Job drawing, mm, ordinate dimensions from the low corner. One solid piece. Coordinates: 2 decimals unless noted, no trailing zeros. Loops run counter-clockwise (first coordinate to the right, second up) from the corner with the lowest first, then second, coordinate; pieces in that order, holes last. Notation, with made-up numbers: (89, -31) - (112, -31) arc R24 ccw to (112, 4) - close; hole circle Ø4 at (32, 52.25). An arc over 180 degrees is marked (long way). Use a Markdown table: item, result. Add a question column.
1) Band-saw the part on B-B (y = 1.6). Give the cut face in (x, z), plus the area to 3 significant figures.
2) Band-saw the part on A-A (z = 5). Give the cut face in (x, y), plus the area to 3 significant figures.
3) Probe probe 1 along Z at (x, y) = (4.7, 1.3); probe 2 along X at (y, z) = (0.7, 4.25); probe 3 along X at (y, z) = (0.8, 1.5). List the from-to ranges inside material, lowest first. Write a range as [from, to].
4) Drop flat-ended pins along their axis: P1, Ø1, axis at y = 2, z = 8.5, coming from the -X side; P2, Ø2.5, axis at x = 4.7, z = 5, coming from the -Y side. Give the stop position or say it passes through.
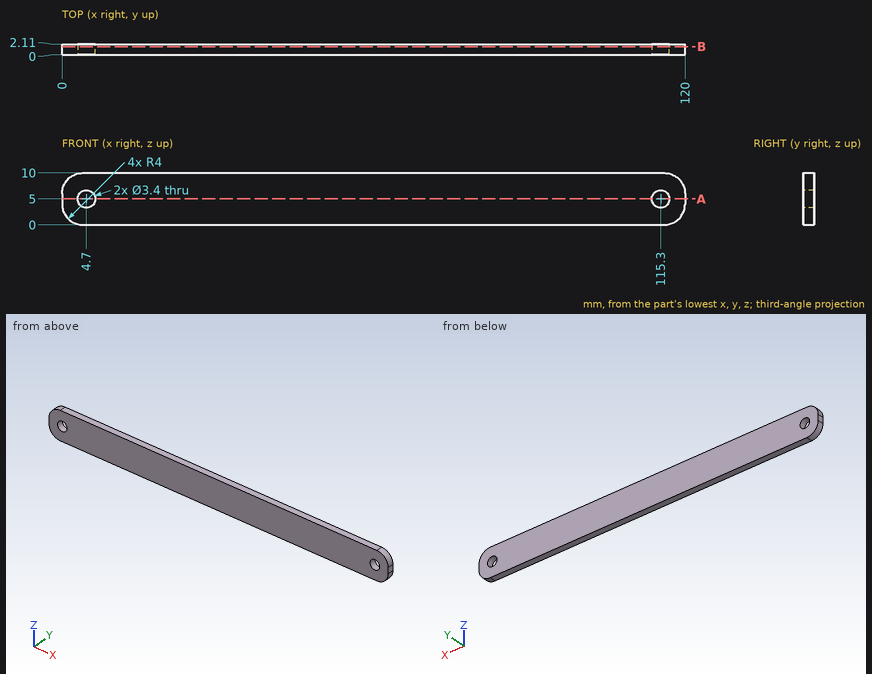
Answer block:
| question | item | result |
|---|---|---|
| 1 | outline | (0, 4) arc R4 ccw to (4, 0) - (116, 0) arc R4 ccw to (120, 4) - (120, 6) arc R4 ccw to (116, 10) - (4, 10) arc R4 ccw to (0, 6) - close; hole circle Ø3.4 at (4.7, 5); hole circle Ø3.4 at (115.3, 5) |
| 1 | area | 1,170 mm2 |
| 2 | outline | (0, 0) - (3, 0) - (3, 2.11) - (0, 2.11) - close; (6.4, 0) - (113.6, 0) - (113.6, 2.11) - (6.4, 2.11) - close; (117, 0) - (120, 0) - (120, 2.11) - (117, 2.11) - close |
| 2 | area | 239 mm2 |
| 3 | probe 1 | [0, 3.3], [6.7, 10] |
| 3 | probe 2 | [0, 3.17], [6.23, 113.77], [116.83, 120] |
| 3 | probe 3 | [0.88, 119.12] |
| 4 | P1 | x = 0.54 |
| 4 | P2 | through |
